Could you check a few things on this model? Use its own coordinates, in mm. A direction names the side the tool comes from. Give positions to 0.01 mm unless a question says otherwise; leave off trailing zeros. Write each loop counter-clockwise with the first axis right and the second up, starting at its lowest first coordinate (ties: lowest second). Pieces come first, ordered by that corner, then holes. Notation, with made-up numbers: (14, 47) - (53, 47) arc R10 ccw to (53, 64) - close; hole circle Ø7 at (13.5, -29). An arc over 180 degrees is marked (long way). Write item = value, one per line.
from build123d import *

# Parameters (mm, degrees)
F0_W     = 107
F0_H     = 41
F1_DEPTH = 24
F3_DEPTH = 48.001
F4_R     = 5
F5_R     = 13
F6_R     = 2.5
F6_R_2   = 5
F7_DEPTH = 41.001
F9_DEPTH = 11


with BuildPart() as f1:
    # F0 (on Front) → F1 (new body, symmetric)
    with BuildSketch(Plane.XZ):
        with Locations((0, 20.5)):
            Rectangle(F0_W, F0_H)
    extrude(amount=F1_DEPTH, both=True)

    # F2 (on face) → F3 (cut, through all)
    with BuildSketch(Plane.XZ.offset(24)):
        with BuildLine():
            ThreePointArc((-27.910571, 11), (0, 30), (27.910571, 11))
            Line((27.910571, 11), (42.5, 11))
            Line((42.5, 11), (42.5, 41))
            Line((42.5, 41), (-53.5, 41))
            Line((-53.5, 41), (-53.5, 11))
            Line((-53.5, 11), (-27.910571, 11))
        make_face()
        with BuildLine():
            Line((-19.05, 0), (19.05, 0))
            ThreePointArc((19.05, 0), (0, 19.05), (-19.05, 0))
        make_face()
    extrude(amount=-F3_DEPTH, mode=Mode.SUBTRACT)

    # F4
    f4_edges = [f1.edges().sort_by_distance(p)[0] for p in [
        (48, -24, 41),
        (48, 24, 41),
    ]]
    fillet(f4_edges, radius=F4_R)

    # F5
    f5_edges = [f1.edges().sort_by_distance(p)[0] for p in [
        (-53.5, -24, 5.5),
        (-53.5, 24, 5.5),
    ]]
    fillet(f5_edges, radius=F5_R)

    # F6 (on Top) → F7 (cut, through all)
    with BuildSketch(Plane.XY):
        Circle(F6_R)
        with Locations((-43, -11)):
            Circle(F6_R_2)
        with Locations((-43, 11)):
            Circle(F6_R_2)
    extrude(amount=F7_DEPTH, mode=Mode.SUBTRACT)

    # F8 (on face) → F9 (cut, through all)
    with BuildSketch(Plane.YZ.offset(53.5)):
        with BuildLine():
            Line((6.5, 41), (-6.5, 41))
            Line((-6.5, 41), (-6.5, 25))
            ThreePointArc((-6.5, 25), (0, 18.5), (6.5, 25))
            Line((6.5, 25), (6.5, 41))
        make_face()
    extrude(amount=-F9_DEPTH, mode=Mode.SUBTRACT)


solid = f1.part
1. If we section it at C-C, the plane z = 38: Please give me the cut outline in (x, y), and give its area (3 significant figures).
Filled sheet:
outline = (42.5, -23.58) - (53.5, -23.58) - (53.5, -6.5) - (42.5, -6.5) - close; (42.5, 6.5) - (53.5, 6.5) - (53.5, 23.58) - (42.5, 23.58) - close
area = 376 mm2
2. For pin 1 (7.5 mm diameter, centred on x = -34.5, y = -2, fed in from +Z); pin 2 (8 mm diameter, centred on x = -43, y = 11, fed in from -Z); pin 3 (15 mm diameter, centred on y = -5.5, z = 20.5, fed in from -X); pin 4 (16 mm diameter, centred on x = 32.5, y = 3.5, fed in from +Z), each with a flat end and sliding along its axis, tell me the tip position at first contact or that it passes through.
Filled sheet:
pin_1 = 11
pin_2 = through
pin_3 = -27.04
pin_4 = 17.31
3. I need wall thicknesses on line 1 (X direction, y = -11, z = 3); line 2 (X direction, y = 9, z = 5); line 3 (Y direction, x = -43, z = 2.5). Which ranges of each line are inside material? Lowest first, please.
Filled sheet:
line_1 = -53.5 to -48, -38 to -18.81, 18.81 to 53.5
line_2 = -53.5 to -47.58, -38.42 to -18.38, 18.38 to 53.5
line_3 = -23.76 to -16, -6 to 6, 16 to 23.76
4. If we section it at B-B, the plane y = 9: Please give me the cut outline in (x, z), and give its area (3 significant figures).
Filled sheet:
outline = (-53.5, 0) - (-47.58, 0) - (-47.58, 11) - (-53.5, 11) - close; (-38.42, 0) - (-19.05, 0) arc R19.05 cw to (19.05, 0) - (53.5, 0) - (53.5, 41) - (42.5, 41) - (42.5, 11) - (27.91, 11) arc R30 ccw to (-27.91, 11) - (-38.42, 11) - close
area = 1,600 mm2
5. Which directions (+Z, -Z, +X, -X, +Y, -Y) give clear straight access to the entire face, cutting with the end or side of a thin tool? Please do faces 1 (the face through (48, -6.5, 33)), 2 (the face through (48, 13, 41)), 3 (the face through (42.5, -6, 19)), 4 (the face through (-41, 0, 11)).
Filled sheet:
face_1 = +Z, +X
face_2 = +Z, +X, -X, +Y, -Y
face_3 = +Z, +Y, -Y
face_4 = +Z, -X, +Y, -Y
6. If we section it at A-A, the plane x = 0: Please give me the cut outline in (y, z).
Filled sheet:
outline = (-24, 19.05) - (-2.5, 19.05) - (-2.5, 30) - (-24, 30) - close; (2.5, 19.05) - (24, 19.05) - (24, 30) - (2.5, 30) - close
7. Thinking about a two-plate mould opening in X: for faces 5 (the face through (48.1, -0.1, 18.5)), 6 (the face through (-0.502, -5.669, 29.996)), 7 (the face through (53.5, 0, 16)), which applies, pulls with the +X half, pulls with the -X half, needs draft (parallel to the pull), parting line crosses it, or undercut?
Filled sheet:
face_5 = needs draft
face_6 = undercut
face_7 = pulls with the +X half
8. If we section it at D-D, the plane x = -43: Please give me the cut outline in (y, z), and give its area (3 significant figures).
Filled sheet:
outline = (-23.76, 0) - (-16, 0) - (-16, 11) - (-23.76, 11) - close; (-6, 0) - (6, 0) - (6, 11) - (-6, 11) - close; (16, 0) - (23.76, 0) - (23.76, 11) - (16, 11) - close
area = 303 mm2
